Geometry check sheet. Reference: drawing and pictorial views, mm from the part's lowest x, y, z. A direction names the side the tool comes from. Round coordinates to 2 decimals unless told otherwise and drop trailing zeros. Write each loop counter-clockwise with the first axis right and the second up, starting at its lowest first coordinate (ties: lowest second). Pieces come first, ordered by that corner, then holes.
Item 1: Section check C-C, the plane x = 53.5. Record the cut outline in (y, z), plus the area to 3 significant figures.
Item 2: Depth check by flat-ended pin: pin 1 (5 mm diameter, centred on x = 26.5, y = 11, fed in from +Z); pin 2 (25 mm diameter, centred on y = 72.5, z = 13, fed in from -X); pin 3 (8 mm diameter, centred on x = 13.5, z = 43.5, fed in from +Y). Enter the tip coordinate at first touch or a pass-through.
Item 3: Material ranges on line 1 along Z through (x, y) = (56.5, 62.5); line 2 along X through (y, z) = (23, 41.5); line 3 along Z through (x, y) = (16, 89.5), recorded low to high.
Item 4: Section check B-B, the plane z = 30. Record the cut outline in (x, y), plus the area to 3 significant figures.
Item 5: Section check D-D, the plane x = 19. Record the cut outline in (y, z).
Item 6: Section check A-A, the plane y = 63. Record the cut outline in (x, z), plus the area to 4 significant figures.
Item 7: Set-up check for the marked faces 1, 2 and 3: record each of +Z, -Z, +X, -X, +Y, -Y from which the full face is reachable in a straight line by a thin tool's end or side.
Item 8: Release check for a two-part mould opening along Y. For the marked faces 4, 5 and 6 record: pulls with the +Y half, pulls with the -Y half, needs draft (parallel to the pull), parting line crosses it, or undercut.
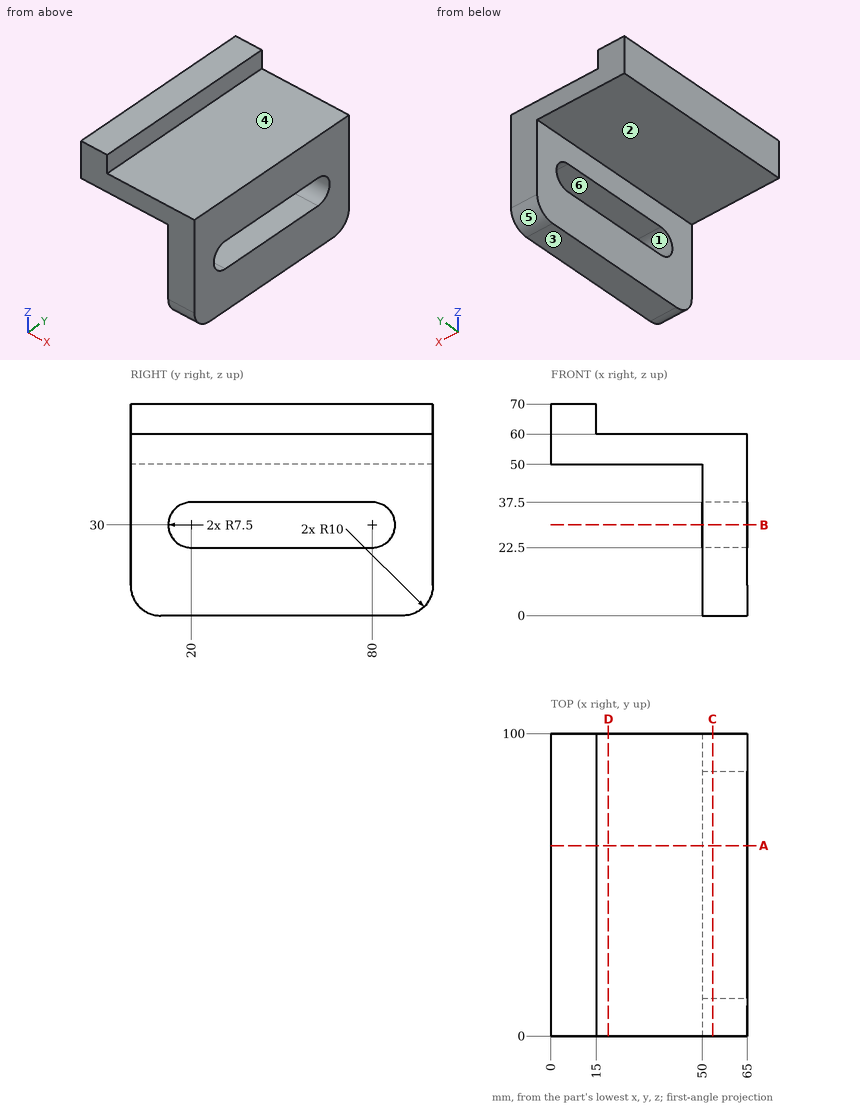
Values found:
1. outline: (0, 10) arc R10 ccw to (10, 0) - (90, 0) arc R10 ccw to (100, 10) - (100, 60) - (0, 60) - close; hole (20, 22.5) - (80, 22.5) arc R7.5 ccw to (80, 37.5) - (20, 37.5) arc R7.5 ccw to start
1. area: 4,880 mm2
2. pin 1: stops at z = 60
2. pin 2: stops at x = 50
2. pin 3: passes through
3. line 1: z = 0 to 22.5, 37.5 to 60
3. line 2: x = 50 to 65
3. line 3: z = 50 to 60
4. outline: (50, 0) - (65, 0) - (65, 12.5) - (50, 12.5) - close; (50, 87.5) - (65, 87.5) - (65, 100) - (50, 100) - close
4. area: 375 mm2
5. outline: (0, 50) - (100, 50) - (100, 60) - (0, 60) - close
6. outline: (0, 50) - (50, 50) - (50, 37.5) - (65, 37.5) - (65, 60) - (15, 60) - (15, 70) - (0, 70) - close; (50, 0) - (65, 0) - (65, 22.5) - (50, 22.5) - close
6. area: 1,325 mm2
7. face 1: +X, -X
7. face 2: -Z, -X, +Y, -Y
7. face 3: -Z, +X, -X, +Y, -Y
8. face 4: needs draft
8. face 5: pulls with the +Y half
8. face 6: undercut
